Check sheet for the modelled part. Datum: model origin and axes. Units: mm. A direction names the side the tool comes from. Give positions to 0.01 mm unless a question says otherwise; leave off trailing zeros. Loops run counter-clockwise (first coordinate to the right, second up) from the corner with the lowest first, then second, coordinate; pieces in that order, holes last. Notation, with made-up numbers: (-28.5, 16) -> (13.5, 16) arc R13 ccw to (13.5, 34) -> close; hole circle Ø6 at (50, 37). An arc over 180 degrees is marked (long way). Write each question's results on one line, items separated by ' | '. Start each with the question number.
Item 1: Gauge pin test, flat ends, axial feed: pin 1 Ø3 at (x, z) = (-1.5, 5.5) entering from -Y; pin 2 Ø1.5 at (x, z) = (2, 4) entering from -Y; pin 3 Ø4 at (x, z) = (-2, 2.5) entering from -Y. Record the tip position at first contact, or that the pin passes through.
Item 2: Cross-section at A-A on z = 4.75. Enter the section's corners in (x, y), then the cut area to 3 significant figures.
Item 3: Mould release check, pull along Z, two halves, no side actions. Record for faces 3 (the face through (-0.59, -4.46, 1.01)), 4 (the face through (0, 0, 8.506)), 5 (the face through (0.65, -1.01, 7.25)): pulls with the +Z half, pulls with the -Z half, needs draft (parallel to the pull), parting line crosses it, or undercut.
Item 4: Access from +Z, -Z, +X, -X, +Y, -Y to the whole of each face (thin tool, end or side, straight path). Record for faces 1 (the face through (2, 0, 2)), 2 (the face through (0, 0, 0)).
Item 5: Scan lines: line 1 along Z through (x, y) = (-2.75, -2.25); line 2 along Y through (x, z) = (0, 3); line 3 along Z through (x, y) = (-1.25, 0). Record each from-to range of solid material in increasing order.
from build123d import *

# Parameters (mm, degrees)
F2_R = 0.5
F3_R = 0.5


with BuildPart() as f1:
    # F0 (on Front) → F1 (revolve)
    with BuildSketch(Plane.XZ):
        Polygon((0, 8.506175), (0, 0), (4.5, 0), (4.5, 2), (1.7, 2), (1.7, 6.5), (1.2, 7), (1.2, 7.5), (1.7, 8), (1.7, 8.5), (1.004275, 8.506175), align=None)
    revolve(axis=Axis((0, 0, 4.253088), (0, 0, -1)))

    # F2
    f2_edges = [f1.edges().sort_by_distance(p)[0] for p in [
        (-1.7, 0, 8.5),
    ]]
    fillet(f2_edges, radius=F2_R)

    # F3
    f3_edges = [f1.edges().sort_by_distance(p)[0] for p in [
        (-4.5, 0, 0),
        (-4.5, 0, 2),
    ]]
    fillet(f3_edges, radius=F3_R)


solid = f1.part
Answer sheet:
1) pin 1: stops at y = -1.7 | pin 2: stops at y = -1.15 | pin 3: stops at y = -4.49
2) outline: circle Ø3.4 at (0, 0) | area: 9.08 mm²
3) face 3: needs draft | face 4: pulls with the +Z half | face 5: undercut
4) face 1: +Z | face 2: -Z, +X, -X, +Y, -Y
5) line 1: z = 0 to 2 | line 2: y = -1.7 to 1.7 | line 3: z = 0 to 6.95, 7.55 to 8.5
